from build123d import *

# Parameters (mm, degrees)
SKETCH1_W           = 170
SKETCH1_H           = 120
BOSS_EXTRUDE1_DEPTH = 90
SKETCH5_R           = 40
BOSS_EXTRUDE3_DEPTH = 160
SKETCH7_R           = 5
BOSS_EXTRUDE4_DEPTH = 50
SKETCH8_R           = 180
BOSS_EXTRUDE5_DEPTH = 80


with BuildPart() as part:
    # Sketch1 → Boss-Extrude1 (new body)
    with BuildSketch(Plane(origin=(0, 0, 0), x_dir=(0, 0, -1), z_dir=(1, 0, 0))):
        with Locations((85, 60)):
            Rectangle(SKETCH1_W, SKETCH1_H)
    extrude(amount=BOSS_EXTRUDE1_DEPTH)

    # Sketch5 → Boss-Extrude3 (add)
    with BuildSketch(Plane(origin=(0, 0, -170), x_dir=(-1, 0, 0), z_dir=(0, 0, -1))):
        with Locations((-45, 60)):
            Circle(SKETCH5_R)
    extrude(amount=BOSS_EXTRUDE3_DEPTH)

    # Sketch7 → Boss-Extrude4 (add)
    with BuildSketch(Plane(origin=(90, 0, 0), x_dir=(0, 0, -1), z_dir=(1, 0, 0))):
        with Locations((80, 70)):
            Circle(SKETCH7_R)
    extrude(amount=BOSS_EXTRUDE4_DEPTH)

    # Sketch8 → Boss-Extrude5 (add)
    with BuildSketch(Plane(origin=(140, 0, 0), x_dir=(0, 0, -1), z_dir=(1, 0, 0))):
        with Locations((80, 70)):
            Circle(SKETCH8_R)
    extrude(amount=BOSS_EXTRUDE5_DEPTH)


solid = part.part
Build history of the part. All positions in model axes, mm. A direction names the side the tool comes from. Round coordinates to 2 decimals unless told otherwise and drop trailing zeros. Order: outer loops, then holes, each group sorted by start corner. A loop starts at its lowest first (then second) coordinate and runs counter-clockwise, first axis right, second up. Notation, with made-up numbers: M -31,-3 L 0,-3 A23 cw 0,23 Z; hole C -33,7.25 d5. An arc over 180 degrees is marked long. Use CSV: the item, a comma, the result in double quotes. Start each with the question number.
(1) Cut at D-D on y = 60. List the corners of the cut face in (x, z), then the cut area to 3 significant figures.
(2) Flat gauge pins, fed straight in: P1, Ø8, axis at y = -28, z = -24, coming from the -X side; P2, Ø1.5, axis at x = 48.5, y = 23.5, coming from the +Z side; P3, Ø6, axis at x = 80.5, y = 27, coming from the -Z side; P4, Ø10, axis at y = 21.5, z = -95, coming from the -X side. Where does each tip first touch, or does it go through?
(3) Tool access for faces 1 (the face through (114.65, 68.085, -84.619)), 2 (the face through (23.5, 93.73, -248.88)), 3 (the face through (44, 0, -84)), 4 (the face through (44, 59, 0)), 5 (the face through (0, 61, -84)): list every direction of +Z, -Z, +X, -X, +Y, -Y with a clear straight run to the whole face (end or side of a thin tool).
(4) Cut at B-B on z = -80. List the corners of the cut face in (x, y).
(5) Mould opens along X. For faces 6 (the face through (220, 73, -77)), 7 (the face through (44, 120, -84)), 8 (the face through (14, 32, -170)) say: +X half, -X half, draft (parallel to the pull), parting line (faces both ways), or undercut.
(6) Drill centre lines: probe 1 along X at (y, z) = (111, -164); probe 2 along X at (y, z) = (157.5, -132); probe 3 along Y at (x, z) = (198, -237.5). Where is each one in solid material? Low to high.
(7) Cut at C-C on x = 45. List the corners of the cut face in (y, z).
(8) Cut at A-A on y = 109.5. List the corners of the cut face in (x, z).
Findings:
1,outline,"M 0,-170 L 5,-170 L 5,-330 L 85,-330 L 85,-170 L 90,-170 L 90,0 L 0,0 Z; M 140,-259.72 L 220,-259.72 L 220,99.72 L 140,99.72 Z"
1,area,"56,900 mm^2"
2,P1,"stops at x = 140"
2,P2,"stops at z = 0"
2,P3,"stops at z = -170"
2,P4,"stops at x = 0"
3,face 1,"none"
3,face 2,"-Z"
3,face 3,"+Z, -Z, -X, -Y"
3,face 4,"+Z, -X, +Y, -Y"
3,face 5,"+Z, -Z, -X, +Y, -Y"
4,outline,"M 0,0 L 90,0 L 90,65 L 140,65 L 140,-110 L 220,-110 L 220,250 L 140,250 L 140,75 L 90,75 L 90,120 L 0,120 Z"
5,face 6,"+X half"
5,face 7,"draft"
5,face 8,"undercut"
6,probe 1,"x = 0 to 90, 140 to 220"
6,probe 2,"x = 140 to 220"
6,probe 3,"y = -17.14 to 157.14"
7,outline,"M 0,-170 L 20,-170 L 20,-330 L 100,-330 L 100,-170 L 120,-170 L 120,0 L 0,0 Z"
8,outline,"M 0,-170 L 90,-170 L 90,0 L 0,0 Z; M 140,-255.61 L 220,-255.61 L 220,95.61 L 140,95.61 Z"
